The listing builds one solid part. Answer for the finished solid, in the listing's coordinates (mm). A direction names the side the tool comes from. Round coordinates to 2 decimals unless told otherwise and drop trailing zeros. Loops run counter-clockwise (first coordinate to the right, second up) from the corner with the lowest first, then second, coordinate; pieces in that order, holes last. Notation, with made-up numbers: M -14.5,74.5 L -0.5,74.5 A11 ccw -0.5,87.5 Z; hole C 88.25,86.25 d6. An arc over 180 degrees is marked long. Put each result on its own line as item: value. Start each with the question number.
(1) Section A-A, the plane x = -8.5 is taken. Determine the outline of the cut face in (y, z), then the cut area to 3 significant figures.
(2) Straight lines are drawn through the part: line 1 (Y direction, x = -9.5, z = 0.85); line 2 (Y direction, x = 1.5, z = 1.4); line 3 (Y direction, x = -2, z = 1.5). For each, find the intervals that lie inside material, in ascending order.
(3) Section B-B, the plane y = 13 is taken. Determine the outline of the cut face in (x, z).
(4) Section C-C, the plane x = 7 is taken. Determine the outline of the cut face in (y, z), then the cut area to 3 significant figures.
(5) Flat-ended cylindrical pins translate along their axes: P1, Ø0.8, axis at x = -15, z = 0.5, coming from the -Y side; P2, Ø0.6, axis at x = 2.5, z = 1, coming from the +Y side; P3, Ø0.6, axis at x = -2.5, z = 1.5, coming from the +Y side. Find the tip coordinate at first contact, or state that the pin passes through.
(6) Determine the mould class of faces 6 (the face through (-9, 2.143, 1)), 7 (the face through (-23.03, -1.27, 1.4)), 8 (the face through (-2, 4.281, 1)) for opening direction Y: released by +Y, released by -Y, zero draft, split by the parting line, or undercut.
(7) Which of the six approach directions +Z, -Z, +X, -X, +Y, -Y give full straight-line access (tool end or side, diameter ignored) to faces 1 (the face through (-4.08, 4.74, 1.11)), 2 (the face through (-9, -1.977, 1)), 3 (the face through (2, 5.423, 1)), 4 (the face through (-10, 1, 0.55)), 5 (the face through (-9, -2.577, 1))?
```python
from build123d import *

# Parameters (mm, degrees)
F1_DEPTH = 1.7
F3_DEPTH = 1.15
F5_DEPTH = 1.15
F7_DEPTH = 25
F9_DEPTH = 0.5


with BuildPart() as f1:
    # F0 (on Top) → F1 (new body)
    with BuildSketch(Plane.XY):
        Polygon((3.5258802325, 7.7773156599), (3.5258802325, 5.4234246183), (-20.5959625565, 5.4234246183), (-24.4741197675, 0), (-21.5398941726, -2.5765753817), (3.5258802325, -2.5765753817), (3.563464143, -4.7479634116), (14.9142147576, -6.0714449676), (22.6833798525, -15.7455861511), (34.9059272557, -15.9271247482), (42.5230842084, -8.8459979743), (42.5230842084, 0.111364905), (42.5323378295, 9.0101445094), (34.9059272557, 17.2138623893), (23.4355190769, 17.2138623893), (14.9758500308, 10.5328802019), align=None)
    extrude(amount=F1_DEPTH)

    # F2 (on face) → F3 (cut)
    with BuildSketch(Plane(origin=(0, 0, 0), x_dir=(1, 0, 0), z_dir=(0, 0, -1))):
        Polygon((-24.1591534096, 0.2765753817), (4.3114135042, 0.2765753817), (3.8650040515, 1.9765753817), (-22.2231791909, 1.9765753817), align=None)
        Polygon((-26.6171693802, 0.2765753817), (-24.1591534096, 0.2765753817), (-22.2231791909, 1.9765753817), (-25.9880051017, 1.9765753817), align=None)
    extrude(amount=-F3_DEPTH, mode=Mode.SUBTRACT)

    # F4 (on face) → F5 (cut)
    with BuildSketch(Plane.XY.offset(1.7)):
        Polygon((5.3927684203, 2.1434246183), (-25.6233029068, 2.1434246183), (-26.0389186442, 0.5034246183), (5.3698872216, 0.5034246183), align=None)
    extrude(amount=-F5_DEPTH, mode=Mode.SUBTRACT)

    # F6 (on face) → F7 (cut)
    with BuildSketch(Plane.XY.offset(1.7)):
        Polygon((-5.3833839484, 6.7872931249), (-0.3340959956, 5.4234246183), (0, 7.7773156599), (-22.1384502947, 7.9461717978), (-23.2389890977, 4.8430952587), (-21.9463394889, 3.5349845421), (-20.9003388882, 6.0035409406), align=None)
        Polygon((-1.5771881219, 4.2808800936), (-0.3340959956, 5.4234246183), (-20.5959625565, 5.4234246183), (-21.9463394889, 3.5349845421), (-21.7945538461, 3.5349845421), (-21.1666878313, 4.1554295458), (-20.8302091438, 4.2808800936), (-20.3477170239, 4.2808800936), (-20.2410556376, 4.3186801486), (-19.5979364216, 4.9228575081), (-19.3608161062, 4.9228575081), (-19.184730947, 5.074087996), (-18.6641020609, 5.074087996), (-18.2254650205, 4.9228575081), (-16.9939434519, 4.8885419965), (-16.5155499687, 4.9228575081), (-15.9821361303, 5.2939280868), (-15.3820421547, 5.2939280868), (-14.1877273184, 4.8885419965), (-12.4018825591, 4.8885419965), (-10.6601839463, 3.6888930481), (-9.1968299821, 3.6888930481), (-7.4136951007, 5.1924162544), (-4.8006242141, 5.1924162544), (-3.3421660773, 4.2808800936), align=None)
    extrude(amount=-F7_DEPTH, mode=Mode.SUBTRACT)

    # F8 (on face) → F9 (cut)
    with BuildSketch(Plane(origin=(0, 0, 0), x_dir=(1, 0, 0), z_dir=(0, 0, -1))):
        Polygon((4.9785347655, -5.9697870165), (4.9301558991, -2.4234246183), (-25.2411490917, -2.4234246183), (-25.5858246237, -5.4234246183), align=None)
    extrude(amount=-F9_DEPTH, mode=Mode.SUBTRACT)


solid = f1.part
```
Recorded:
1. outline: M -2.58,0 L -1.98,0 L -1.98,1.15 L -0.28,1.15 L -0.28,0 L 2.42,0 L 2.42,0.5 L 4.28,0.5 L 4.28,1.7 L 2.14,1.7 L 2.14,0.55 L 0.5,0.55 L 0.5,1.7 L -2.58,1.7 Z
1. area: 6.88 mm²
2. line 1: y = -2.58 to -1.98, -0.28 to 0.5, 2.14 to 3.69
2. line 2: y = -2.58 to 0.5, 2.14 to 5.42
2. line 3: y = -2.58 to 0.5, 2.14 to 4.28
3. outline: M 18.1,0 L 38.82,0 L 38.82,1.7 L 18.1,1.7 Z
4. outline: M -5.15,0 L 8.61,0 L 8.61,1.7 L -5.15,1.7 Z
4. area: 23.4 mm²
5. P1: stops at y = -2.58
5. P2: stops at y = 5.42
5. P3: stops at y = 4.28
6. face 6: undercut
6. face 7: released by -Y
6. face 8: released by +Y
7. face 1: +Z, -Z, +Y
7. face 2: -Z, -X
7. face 3: +Z, -Z, -X, +Y
7. face 4: +Z, -X
7. face 5: +Z, -Z, -X, -Y
